The drawing under review shows one solid part. Ordinate dimensions are in mm from its lowest x, y, z. Coordinates: 2 decimals unless noted, no trailing zeros. Write each loop counter-clockwise with the first axis right and the second up, starting at its lowest first coordinate (ties: lowest second). Pieces come first, ordered by that corner, then holes.
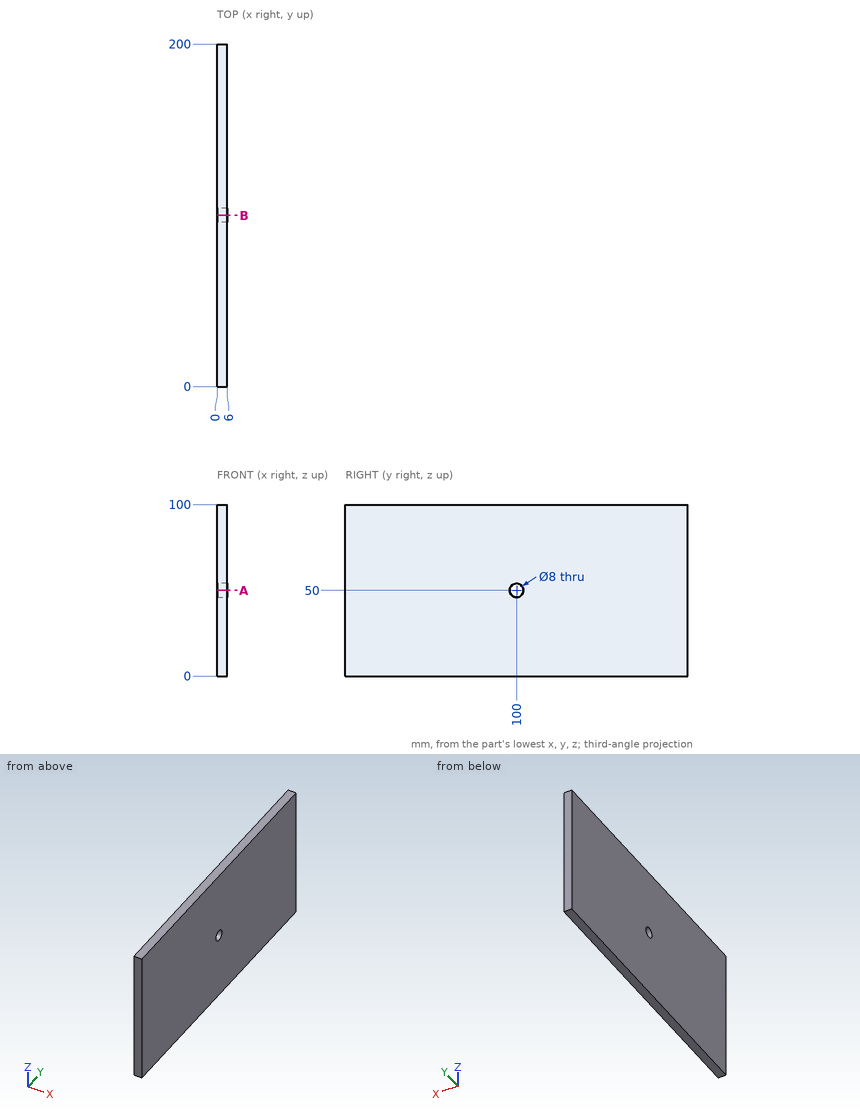
1) Consider section B-B (y = 100). Give the boundary of the cut face in (x, z).
2) Consider section A-A (z = 50). Give the boundary of the cut face in (x, y).
3) For L1, parallel to Z at x = 1.3, y = 100; L2, parallel to Y at x = 4.15, z = 50; L3, parallel to Y at x = 3.6, z = 52.5, list the stretches that pass through material, from the lowest coordinate up.
Results:
1. outline: (0, 0) - (6, 0) - (6, 46) - (0, 46) - close; (0, 54) - (6, 54) - (6, 100) - (0, 100) - close
2. outline: (0, 0) - (6, 0) - (6, 96) - (0, 96) - close; (0, 104) - (6, 104) - (6, 200) - (0, 200) - close
3. L1: z = 0 to 46, 54 to 100
3. L2: y = 0 to 96, 104 to 200
3. L3: y = 0 to 96.88, 103.12 to 200
